CAD build for the part. Positions are in the model's coordinates, mm. A direction names the side the tool comes from. Round coordinates to 2 decimals unless told otherwise and drop trailing zeros. Loops run counter-clockwise (first coordinate to the right, second up) from the corner with the lowest first, then second, coordinate; pieces in that order, holes last.
```python
from build123d import *

# Parameters (mm, degrees)
BOSS_EXTRUDE1_DEPTH     = 8
BOSS_EXTRUDE2_DEPTH     = 4
BOSS_EXTRUDE3_DEPTH     = 2
SKETCH4_R               = 1.6
CUT_EXTRUDE1_DEPTH      = 12
CUT_EXTRUDE1_DEPTH_BACK = 59.38298604
SKETCH5_R               = 3.149940151
CUT_EXTRUDE2_DEPTH      = 10
SKETCH5_2_R             = 3.149940151
CUT_EXTRUDE3_DEPTH      = 9


with BuildPart() as part:
    # Sketch1 → Boss-Extrude1 (new body)
    with BuildSketch(Plane(origin=(0, 0, 0), x_dir=(0, 0, -1), z_dir=(1, 0, 0))):
        Polygon((-74.695832275, 27.991563326), (-71.872967623, 35.747320216), (73.384955245, -24.208131169), (74.695832275, -35.747320216), (66.050660164, -32.600734897), (69.060437425, -24.331439834), align=None)
    extrude(amount=BOSS_EXTRUDE1_DEPTH)

    # Sketch2 → Boss-Extrude2 (add)
    with BuildSketch(Plane.ZY):
        Polygon((74.695832275, 27.991563326), (63.419520826, 23.887321606), (60.770717842, 31.164847991), (71.872967623, 35.747320216), align=None)
    extrude(amount=BOSS_EXTRUDE2_DEPTH)

    # Sketch6 → Boss-Extrude3 (add)
    with BuildSketch(Plane.ZY):
        Polygon((-74.695832275, -35.747320216), (-66.050660164, -32.600734897), (-69.060437425, -24.331439834), (-69.733422771, -22.700955013), (-73.384955245, -24.208131169), (-73.586089176, -25.978642362), align=None)
    extrude(amount=BOSS_EXTRUDE3_DEPTH)

    # Sketch4 → Cut-Extrude1 (cut, two sides)
    with BuildSketch(Plane(origin=(0, 0.710394692, -0.258562522), x_dir=(-1, 0, 0), z_dir=(0, -0.939692621, 0.342020143))) as cut_extrude1_sk:
        with Locations((-2.394217395, -73.485294271)):
            Circle(SKETCH4_R)
        with Locations((-2.394217395, 77.00491749)):
            Circle(SKETCH4_R)
    extrude(amount=CUT_EXTRUDE1_DEPTH, mode=Mode.SUBTRACT)
    extrude(cut_extrude1_sk.sketch, amount=-CUT_EXTRUDE1_DEPTH_BACK, mode=Mode.SUBTRACT)

    # Sketch5 → Cut-Extrude2 (cut)
    with BuildSketch(Plane(origin=(0, 5.408857796, -1.968663239), x_dir=(-1, 0, 0), z_dir=(0, -0.939692621, 0.342020143))):
        with Locations((-2.394217395, -73.485294271)):
            Circle(SKETCH5_R)
        with Locations((-2.394217395, 77.514705729)):
            Circle(SKETCH5_R)
    extrude(amount=-CUT_EXTRUDE2_DEPTH, mode=Mode.SUBTRACT)

    # Sketch5_2 → Cut-Extrude3 (cut)
    with BuildSketch(Plane(origin=(0, 5.408857796, -1.968663239), x_dir=(-1, 0, 0), z_dir=(0, -0.939692621, 0.342020143))):
        with Locations((-2.394217395, -73.485294271)):
            Circle(SKETCH5_2_R)
        with Locations((-2.394217395, 77.514705729)):
            Circle(SKETCH5_2_R)
    extrude(amount=CUT_EXTRUDE3_DEPTH, mode=Mode.SUBTRACT)


solid = part.part
```
Item 1: Probe line 1 (Z direction, x = 3, y = 32); line 2 (X direction, y = -13.5, z = -40); line 3 (Y direction, x = 1.75, z = 62). List the from-to ranges inside material, lowest first.
Answers follow:
line 1: z = 62.79 to 63.26, 69.84 to 73.24
line 2: x = 0 to 8
line 3: y = 23.37 to 31.67
Item 2: 3-axis set-ups, long thin cutter, end or side, ignore diameter. For faces 4 (the flat face through (2.44, -30.11, -73.24)), 5 (the flat face through (-4, 30, 68)), 6 (the flat face through (-1.97, 27.48, 62.11)), 7 (the flat face through (3.07, -28.524, -67.534)): which of +Z, -Z, +X, -X, +Y, -Y reach the whole face in a straight line?
Answers follow:
face 4: none
face 5: +Z, -Z, -X, +Y, -Y
face 6: -Z, -X, -Y
face 7: +Z, +X, -X
Item 3: Cut at A-A, the plane y = -3.5. Give the cut face in (x, z).
Answers follow:
outline: (0, -23.21) - (8, -23.21) - (8, -11.83) - (0, -11.83) - close
Item 4: Flat gauge pins, fed straight in: P1, Ø7, axis at y = -27.5, z = -70.5, coming from the -X side; P2, Ø12, axis at y = 22, z = 22, coming from the -X side; P3, Ø4, axis at x = -1.5, z = -14.5, coming from the -Y side. Where does each tip first touch, or does it go through?
Answers follow:
P1: stops at x = -2
P2: passes through
P3: stops at y = -4.95
Item 5: Two-plate mould, pull along Z, no slides. Class faces 1 (the cylindrical face through (1.656, -31.124, -69.108)), 2 (the flat face through (2.084, 31.924, 73.265)), 3 (the flat face through (-2, -29, -70)): released by +Z, released by -Z, zero draft, split by the parting line, or undercut.
Answers follow:
face 1: undercut
face 2: released by +Z
face 3: zero draft
Item 6: Cut at B-B, the plane z = 3. Give the cut face in (x, y).
Answers follow:
outline: (0, 1.9) - (8, 1.9) - (8, 7.32) - (0, 7.32) - close
